Autodesk Inventor part; units mm, degrees
ref_plane "YZ Plane" through (0, 0, 0) normal (1, 0, 0) x (0, 1, 0)
ref_plane "XZ Plane" through (0, 0, 0) normal (0, 1, 0) x (-1, 0, 0)
ref_plane "XY Plane" through (0, 0, 0) normal (0, 0, 1) x (1, 0, 0)
sketch "Sketch1" plane through (0, 0, 0) normal (0, 0, 1) x (1, 0, 0)
  circle A0 centre (0, 0) radius 47.625
  line L0 (0, 0) -> (21.4313, 37.12)
  line L1 (0, 0) -> (42.8625, 0) construction
  circle A1 centre (21.4313, 37.12) radius 1.8415
  circle A2 centre (-21.4312, 37.12) radius 1.8415
  circle A3 centre (-42.8625, 0) radius 1.8415
  circle A4 centre (-21.4313, -37.12) radius 1.8415
  circle A5 centre (21.4312, -37.12) radius 1.8415
  circle A6 centre (42.8625, 0) radius 1.8415
  dimension "d0" = 95.25
  dimension "d1" = 42.8625
  dimension "d2" = 60
  dimension "d3" = 3.683
  dimension "d6" = 360
extrude "Extrusion1" add sketch "Sketch1" along normal blind 3.175
sketch "Sketch3" plane through (0, 0, 0) normal (0, 0, -1) x (-1, 0, 0)
  circle A0 centre (0, 0) radius 41.275
  circle A1 centre (0, 0) radius 34.544
  dimension "d10" = 82.55
  dimension "d11" = 69.088
extrude "Extrusion2" add sketch "Sketch3" along normal blind 1.5875 contours A1
sketch "Sketch6" plane through (0, 0, -1.5875) normal (0, 0, -1) x (-1, 0, 0)
  circle A0 centre (0, 0) radius 33.02
  dimension "d27" = 66.04
extrude "Extrusion4" cut sketch "Sketch6" against normal blind 25.4
sketch "Sketch8" plane through (0, 0, 3.175) normal (0, 0, 1) x (1, 0, 0)
  line L0 (0, 0) -> (39.3779, 10.5513)
  line L1 (0, 0) -> (40.767, 0) construction
  circle A0 centre (39.3779, 10.5513) radius 2.54
  line L2 (0, 0) -> (0, 8.7749)
  circle A1 centre (39.3779, -10.5513) radius 2.54
  circle A2 centre (-39.3779, 10.5513) radius 2.54
  circle A3 centre (-39.3779, -10.5513) radius 2.54
  circle A4 centre (21.4313, 37.12) radius 1.8415
  line L3 (21.4313, 37.12) -> (0, 0)
  circle A5 centre (28.8266, 28.8266) radius 2.54
  line L4 (28.8266, 28.8266) -> (0, 0)
  circle A6 centre (-28.8266, 28.8266) radius 2.54
  dimension "d30" = 40.767
  dimension "d31" = 15
  dimension "d32" = 5.08
  dimension "d35" = 15
  dimension "d36" = 40.767
  dimension "d37" = 5.08
extrude "Extrusion5" cut sketch "Sketch8" against normal blind 25.4 contours A0 | A1 | A2 | A3
extrude "Extrusion6" cut sketch "Sketch8" against normal blind 25.4 contours A5 | A6
sketch "Sketch10" plane through (0, 0, 3.175) normal (0, 0, 1) x (1, 0, 0)
  line L0 (0, 0) -> (-13.8997, 38.1891) construction
  line L1 (0, 0) -> (40.64, 0) construction
  circle A0 centre (-13.8997, 38.1891) radius 2.8575
  dimension "d44" = 40.64
  dimension "d45" = 110
  dimension "d46" = 5.715
extrude "Extrusion8" cut sketch "Sketch10" against normal through all
sketch "Sketch9" plane through (0, 0, 3.175) normal (0, 0, 1) x (1, 0, 0)
  circle A0 centre (0, 0) radius 47.625
  circle A1 centre (0, 0) radius 47.117
  dimension "d40" = 95.25
  dimension "d41" = 94.234
extrude "PRINT_FEATURE_1" [suppressed]
equation "\"d35\" = d31"
equation "\"d36\" = d30"
equation "\"d37\" = d32"
properties part number "forwardBallastSealingWallRear" material "ABS Plastic"
Source: CAD feature listing. Evaluate the final solid. Frame: model axes, mm. A direction names the side the tool comes from. Coordinates: 2 decimals unless noted, no trailing zeros. Loops run counter-clockwise (first coordinate to the right, second up) from the corner with the lowest first, then second, coordinate; pieces in that order, holes last. Notation, with made-up numbers: (18.25, 62.25) -> (70.25, 62.25) arc R25 ccw to (70.25, 81.25) -> close; hole circle Ø1 at (3, 27.25). An arc over 180 degrees is marked (long way). Answer in a Markdown table with one row per item. Add a question column.
Q1. Pull-direction query (X, two-part tool) for faces 3 (the face through (-41.915, -10.44, 1.61)), 4 (the face through (-37.794, 28.979, 1.565)), 5 (the face through (-32, -10, 3.175)), 6 (the face through (-29.157, 31.345, 1.61)); classes: pulls with the +X half, pulls with the -X half, needs draft (parallel to the pull), parting line crosses it, or undercut.
Q2. Section D-D on y = -37.12. Return the cut outline in (x, z) (3 decimals).
Q3. Section A-A on x = 0. Return the cut outline in (y, z) (1 decimal), and give its area (3 significant figures).
Q4. Ray query, line 1 along Y through (x, z) = (0, 1.75) (3 decimals); line 2 along X through (y, z) = (10.5, 1.9); line 3 along Y through (x, z) = (-28.5, 1.5). Return the intervals inside material, ascending.
Q5. Section C-C on z = 2.3. Give the number of separate pieces and of enclosed holes in the cut face, and give its area (3 significant figures).
Q6. Section B-B on y = 0. Return the cut outline in (x, z) (1 decimal), and give its area (3 significant figures).
Q7. Contact query for flat-ended pins moving along their axis: pin 1 Ø4 at (x, y) = (21.43, -37.12) entering from -Z; pin 2 Ø2 at (x, z) = (-32.5, -0.5) entering from -Y; pin 3 Ø1.5 at (y, z) = (8.5, 2.5) entering from -X. Output: stop coordinate, or through.
Q8. Reachability of faces 1 (the face through (41.724, 9.578, 1.61)), 2 (the face through (32, 14, 0)) from +Z, -Z, +X, -X, +Y, -Y: full face, straight path, thin tool, end or side. Return the list, or none.
Computed values:
| question | item | result |
|---|---|---|
| 1 | face 3 | undercut |
| 1 | face 4 | parting line crosses it |
| 1 | face 5 | needs draft |
| 1 | face 6 | undercut |
| 2 | outline | (-29.837, 0) -> (-23.273, 0) -> (-23.273, 3.175) -> (-29.837, 3.175) -> close; (-19.59, 0) -> (19.59, 0) -> (19.59, 3.175) -> (-19.59, 3.175) -> close; (23.273, 0) -> (29.837, 0) -> (29.837, 3.175) -> (23.273, 3.175) -> close |
| 3 | outline | (-47.6, 0) -> (-34.5, 0) -> (-34.5, -1.6) -> (-33, -1.6) -> (-33, 3.2) -> (-47.6, 3.2) -> close; (33, -1.6) -> (34.5, -1.6) -> (34.5, 0) -> (47.6, 0) -> (47.6, 3.2) -> (33, 3.2) -> close |
| 3 | area | 97.6 mm^2 |
| 4 | line 1 | y = -47.625 to -33.02, 33.02 to 47.625 |
| 4 | line 2 | x = -46.45 to -41.92, -36.84 to -31.31, 31.31 to 36.84, 41.92 to 46.45 |
| 4 | line 3 | y = -38.16 to -16.68, 16.68 to 26.31, 31.35 to 38.16 |
| 5 | separate pieces | 1 |
| 5 | enclosed holes | 14 |
| 5 | area | 3,490 mm^2 |
| 6 | outline | (-47.6, 0) -> (-44.7, 0) -> (-44.7, 3.2) -> (-47.6, 3.2) -> close; (-41, 0) -> (-34.5, 0) -> (-34.5, -1.6) -> (-33, -1.6) -> (-33, 3.2) -> (-41, 3.2) -> close; (33, -1.6) -> (34.5, -1.6) -> (34.5, 0) -> (41, 0) -> (41, 3.2) -> (33, 3.2) -> close; (44.7, 0) -> (47.6, 0) -> (47.6, 3.2) -> (44.7, 3.2) -> close |
| 6 | area | 74.2 mm^2 |
| 7 | pin 1 | stops at z = 0 |
| 7 | pin 2 | stops at y = -35.6 |
| 7 | pin 3 | stops at x = -46.99 |
| 8 | face 1 | +Z, -Z |
| 8 | face 2 | -Z |
